Here's how the part is built. I have some questions about the finished solid (model axes, mm). Give positions to 0.01 mm unless a question says otherwise; leave off trailing zeros. Write each loop counter-clockwise with the first axis right and the second up, starting at its lowest first coordinate (ties: lowest second). Pieces come first, ordered by that corner, then holes. Notation, with made-up numbers: M 22.5,38 L 65.5,38 A27 ccw 65.5,75 Z; hole C -21,12.25 d1. An arc over 180 degrees is marked long. Answer as CSV lines item,"result". Start each with the question number.
Q1. Suppose I cut it at A-A (z = 2.55). Write out the boundary of the cut face in (x, y).
Q2. If I drill on line 1 along X through (y, z) = (1.25, 1.3); line 2 along Y through (x, z) = (-16, 2.95); line 3 along Y through (x, z) = (-7.5, 3.75), over which ranges is the centre line in solid material (lowest first)?
Q3. Suppose I cut it at C-C (y = -0.5). Write out the boundary of the cut face in (x, z).
Q4. Thinking about a two-plate mould opening in X: for faces 1 (the cylindrical face through (-19.615, 0.092, 1.972)), 2 (the flat face through (0, 0, 0)), which applies, +X half, -X half, draft (parallel to the pull), parting line (faces both ways), or undercut?
Q5. Suppose I cut it at B-B (y = 3). Write out the boundary of the cut face in (x, z).
Q6. Suppose I cut it at D-D (x = -8). Write out the boundary of the cut face in (y, z), then the cut area to 3 significant figures.
```python
from build123d import *

# Parameters (mm, degrees)
F0_R     = 2.1
F0_R_2   = 1.65
F1_DEPTH = 4


with BuildPart() as f1:
    # F0 (on Top) → F1 (new body)
    with BuildSketch(Plane.XY):
        with BuildLine():
            ThreePointArc((-14.95, -4), (-0.083435, -1.499923), (14.783129, -4))
            ThreePointArc((14.783129, -4), (17.612798, -4.585324), (20.441514, -3.995413))
            ThreePointArc((20.441514, -3.995413), (22.749633, -2.382687), (24.25, 0))
            ThreePointArc((24.25, 0), (22.695398, 2.39643), (20.3309, 3.999182))
            ThreePointArc((20.3309, 3.999182), (17.557097, 4.555734), (14.783129, 4))
            ThreePointArc((14.783129, 4), (-0.083435, 1.499923), (-14.95, 4))
            ThreePointArc((-14.95, 4), (-17.606941, 4.512271), (-20.263877, 3.999976))
            ThreePointArc((-20.263877, 3.999976), (-22.668799, 2.410422), (-24.25, 0))
            ThreePointArc((-24.25, 0), (-20.422404, -3.91209), (-14.95, -4))
        make_face()
        with Locations((-17.516871, 0)):
            Circle(F0_R, mode=Mode.SUBTRACT)
        with Locations((17.483129, 0)):
            Circle(F0_R_2, mode=Mode.SUBTRACT)
    extrude(amount=F1_DEPTH)


solid = f1.part
```
Resolved:
1,outline,"M -24.25,0 A7.2 ccw -14.95,-4 A45.45 cw 14.78,-4 A7.1 ccw 20.44,-4 A7.1 ccw 24.25,0 A7.2 ccw 20.33,4 A7.2 ccw 14.78,4 A45.45 cw -14.95,4 A7.15 ccw -20.26,4 A7.15 ccw Z; hole C -17.52,0 d4.2; hole C 17.48,0 d3.3"
2,line 1,"-23.61 to -19.2, -15.83 to 16.41, 18.56 to 23.61"
2,line 2,"-4.32 to -1.45, 1.45 to 4.33"
2,line 3,"-2.11 to 2.11"
3,outline,"M -24.03,0 L -19.56,0 L -19.56,4 L -24.03,4 Z; M -15.48,0 L 15.91,0 L 15.91,4 L -15.48,4 Z; M 19.06,0 L 24.04,0 L 24.04,4 L 19.06,4 Z"
4,face 1,"undercut"
4,face 2,"draft"
5,outline,"M -22,0 L -11.66,0 L -11.66,4 L -22,4 Z; M 11.5,0 L 22.02,0 L 22.02,4 L 11.5,4 Z"
6,outline,"M -2.19,0 L 2.19,0 L 2.19,4 L -2.19,4 Z"
6,area,"17.6 mm^2"
